Design review of the part built by this model. Coordinates are the model's own, in mm. A direction names the side the tool comes from. Coordinates: 2 decimals unless noted, no trailing zeros. Write each loop counter-clockwise with the first axis right and the second up, starting at its lowest first coordinate (ties: lowest second). Pieces come first, ordered by that corner, then holes.
```python
from build123d import *

# Parameters (mm, degrees)
F0_W     = 18
F0_H     = 6
F1_DEPTH = 6
F2_R     = 1.5
F3_DEPTH = 10
F5_DEPTH = 25
F6_R     = 2


with BuildPart() as f1:
    # F0 (on Top) → F1 (new body)
    with BuildSketch(Plane.XY):
        with Locations((6, 0)):
            Rectangle(F0_W, F0_H)
    extrude(amount=F1_DEPTH)

    # F2 (on face) → F3 (cut)
    with BuildSketch(Plane.XY.offset(6)):
        Circle(F2_R)
    extrude(amount=-F3_DEPTH, mode=Mode.SUBTRACT)

    # F4 (on face) → F5 (cut)
    with BuildSketch(Plane.XY.offset(6)):
        with BuildLine():
            Line((3.708099, 1.5), (15, 1.5))
            Line((15, 1.5), (15, 3))
            Line((15, 3), (2.645751, 3))
            ThreePointArc((2.645751, 3), (3.264254, 2.311849), (3.708099, 1.5))
        make_face()
        with BuildLine():
            Line((15, -3), (15, -1.5))
            Line((15, -1.5), (3.708099, -1.5))
            ThreePointArc((3.708099, -1.5), (3.264254, -2.311849), (2.645751, -3))
            Line((2.645751, -3), (15, -3))
        make_face()
    extrude(amount=-F5_DEPTH, mode=Mode.SUBTRACT)

    # F6
    f6_edges = [f1.edges().sort_by_distance(p)[0] for p in [
        (15, 0, 6),
        (15, 0, 0),
    ]]
    fillet(f6_edges, radius=F6_R)


solid = f1.part
```
(1) Consider section B-B (x = 0). Give the boundary of the cut face in (y, z).
(2) Insertion check: pin 1 Ø3 at (x, z) = (7.5, 3.5) entering from +Y. The pin has a flat end and moves straight along its axis. Give the tip position at first contact, or say it passes through.
(3) Consider section C-C (z = 5.15). Give the boundary of the cut face in (x, y).
(4) Consider section A-A (y = 0). Give the boundary of the cut face in (x, z).
(5) Wall thickness on line 1 (Y direction, x = 0, z = 1.6); line 2 (Y direction, x = 6, z = 5.2); line 3 (X direction, y = -0.5, z = 1.35): over which ranges is each line inside the solid? List them lowest first.
(6) Mouldability with a two-part tool opening along Y and no side actions: class faces 4 (the flat face through (15, 0, 3)), 5 (the flat face through (0, -3, 3)), 6 (the cylindrical face through (-1.5, 0.07, 3.04)) as +Y half, -Y half, draft (parallel to the pull), parting line (faces both ways), or undercut.
(7) For faces 1 (the flat face through (9, 1.5, 3)), 2 (the cylindrical face through (14.4, 0.02, 5.43)), 3 (the flat face through (9, -1.5, 3)), list the 3-axis set-ups (+Z, -Z, +X, -X, +Y, -Y) from which the entire face can be reached by the end or side of a thin tool; tool diameter is ignored.
(8) Consider section D-D (z = 1.55). Give the boundary of the cut face in (x, y).
Results:
1. outline: (-3, 0) - (-1.5, 0) - (-1.5, 6) - (-3, 6) - close; (1.5, 0) - (3, 0) - (3, 6) - (1.5, 6) - close
2. pin 1: stops at y = 1.5
3. outline: (-3, -3) - (2.65, -3) arc R4 ccw to (3.71, -1.5) - (14.64, -1.5) - (14.64, 1.5) - (3.71, 1.5) arc R4 ccw to (2.65, 3) - (-3, 3) - close; hole circle Ø3 at (0, 0)
4. outline: (-3, 0) - (-1.5, 0) - (-1.5, 6) - (-3, 6) - close; (1.5, 0) - (13, 0) arc R2 ccw to (15, 2) - (15, 4) arc R2 ccw to (13, 6) - (1.5, 6) - close
5. line 1: y = -3 to -1.5, 1.5 to 3
5. line 2: y = -1.5 to 1.5
5. line 3: x = -3 to -1.41, 1.41 to 14.89
6. face 4: draft
6. face 5: -Y half
6. face 6: undercut
7. face 1: +Z, -Z, +X, +Y
7. face 2: +Z, +X, +Y, -Y
7. face 3: +Z, -Z, +X, -Y
8. outline: (-3, -3) - (2.65, -3) arc R4 ccw to (3.71, -1.5) - (14.95, -1.5) - (14.95, 1.5) - (3.71, 1.5) arc R4 ccw to (2.65, 3) - (-3, 3) - close; hole circle Ø3 at (0, 0)
